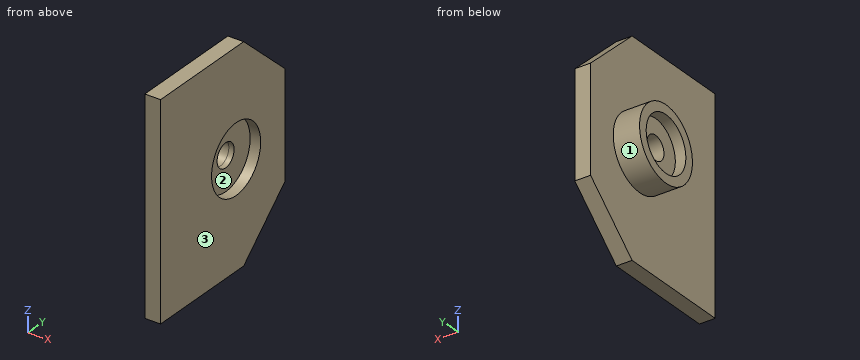
Autodesk Inventor part; units mm, degrees
ref_plane "YZ Plane" through (0, 0, 0) normal (1, 0, 0) x (0, 1, 0)
ref_plane "XZ Plane" through (0, 0, 0) normal (0, 1, 0) x (-1, 0, 0)
ref_plane "XY Plane" through (0, 0, 0) normal (0, 0, 1) x (1, 0, 0)
sketch "Esquisse1" plane through (0, 0, 0) normal (1, 0, 0) x (0, 1, 0)
  circle A0 centre (0, 0) radius 5.25
  circle A1 centre (0, 0) radius 7
  dimension "d0" = 10.5
  dimension "d1" = 14
extrude "Extrusion1" add sketch "Esquisse1" along normal blind 10
sketch "Esquisse2" plane through (10, 0, 0) normal (1, 0, 0) x (0, 0, -1)
  line L0 (20, -20) -> (-20, 20) construction
  line L1 (-20, -20) -> (20, 20) construction
  circle A0 centre (0, 0) radius 17.5 construction
  line L2 (0, 0) -> (0, 13) construction
  line L3 (0, 13) -> (10, 13)
  line L4 (10, 13) -> (-10, 13)
  line L5 (0, 0) -> (0, -20) construction
  line L6 (0, -20) -> (20, -20)
  line L7 (20, -20) -> (-20, -20)
  line L8 (-20, -20) -> (-20, 2)
  line L9 (20, -20) -> (20, 2)
  line L10 (20, 2) -> (10, 13)
  line L11 (-10, 13) -> (-20, 2)
  dimension "d41" = 35
  dimension "d44" = 13
  dimension "d45" = 10
  dimension "d46" = 20
  dimension "d47" = 20
  dimension "d48" = 20
  dimension "d49" = 22
  dimension "d50" = 14.8661
  dimension "d51" = 14.8661
extrude "Extrusion2" add sketch "Esquisse2" along normal blind 3
sketch "Esquisse7" plane through (13, 0, 0) normal (1, 0, 0) x (0, 0, -1)
  circle A0 centre (0, 0) radius 2.25
  dimension "d25" = 4.5
extrude "Extrusion7" cut sketch "Esquisse7" against normal blind 59.75
sketch "Esquisse12" plane through (0, 0, 0) normal (-1, 0, 0) x (0, 0, 1)
  circle A0 centre (0, 0) radius 5.25
  circle A1 centre (0, 0) radius 7
extrude "Extrusion10" cut sketch "Esquisse12" against normal blind 5
sketch "Esquisse13" plane through (13, 0, 0) normal (1, 0, 0) x (0, 0, -1)
  circle A0 centre (0, 0) radius 6.5
  dimension "d52" = 13
extrude "Extrusion11" cut sketch "Esquisse13" against normal blind 2
sketch "Esquisse14" plane through (10, 0, 0) normal (-1, 0, 0) x (0, 0, 1)
  circle A0 centre (0, 0) radius 2.25
  circle A1 centre (0, 0) radius 5.25
extrude "Extrusion12" add sketch "Esquisse14" along normal blind 3
properties part number "percuteur"
Input: part model. Units: mm. Frame: model coordinates. Face numbers are marked on the shaded views. Coordinates: 2 decimals unless noted, no trailing zeros. Write each loop counter-clockwise with the first axis right and the second up, starting at its lowest first coordinate (ties: lowest second). Pieces come first, ordered by that corner, then holes. Notation, with made-up numbers: (-21, -19.5) -> (34, -19.5) arc R18 cw to (34, -12.5) -> close; hole circle Ø10 at (80, 66.25). An arc over 180 degrees is marked (long way). Write each question's results on one line, items separated by ' | '.
Item 1: Section query B-B on x = 12.25. Return loops of the section in (y, z).
Conclusion:
outline: (-20, -20) -> (2, -20) -> (13, -10) -> (13, 10) -> (2, 20) -> (-20, 20) -> close; hole circle Ø13 at (0, 0)
Item 2: Material intervals for probe 1 along Z at (x, y) = (6.3, 0); probe 2 along Y at (x, z) = (12.4, 0); probe 3 along Z at (x, y) = (8.25, 0), sorted ascending.
Conclusion:
probe 1: z = -7 to -5.25, 5.25 to 7 | probe 2: y = -20 to -6.5, 6.5 to 13 | probe 3: z = -7 to -2.25, 2.25 to 7
Item 3: Section query A-A on z = 0. Return loops of the section in (x, y), plus the area to 3 significant figures.
Conclusion:
outline: (5, -7) -> (10, -7) -> (10, -20) -> (13, -20) -> (13, -6.5) -> (11, -6.5) -> (11, -2.25) -> (7, -2.25) -> (7, -5.25) -> (5, -5.25) -> close; (5, 5.25) -> (7, 5.25) -> (7, 2.25) -> (11, 2.25) -> (11, 6.5) -> (13, 6.5) -> (13, 13) -> (10, 13) -> (10, 7) -> (5, 7) -> close | area: 104 mm^2
Item 4: Pin query (flat end, axial travel): pin 1 Ø8 at (y, z) = (2.5, -1) entering from +X; pin 2 Ø3 at (x, z) = (6.5, -0.5) entering from +Y; pin 3 Ø5 at (y, z) = (0, 0) entering from +X; pin 4 Ø5 at (y, z) = (2.5, -1) entering from -X. Return the tip coordinate at first contact, or that it passes through.
Conclusion:
pin 1: stops at x = 13 | pin 2: stops at y = 7 | pin 3: stops at x = 11 | pin 4: stops at x = 7
Item 5: Section query D-D on z = -11. Return loops of the section in (x, y).
Conclusion:
outline: (10, -20) -> (13, -20) -> (13, 11.9) -> (10, 11.9) -> close
Item 6: Section query C-C on y = 0. Return loops of the section in (x, z), plus the area to 3 significant figures.
Conclusion:
outline: (5, -7) -> (10, -7) -> (10, -20) -> (13, -20) -> (13, -6.5) -> (11, -6.5) -> (11, -2.25) -> (7, -2.25) -> (7, -5.25) -> (5, -5.25) -> close; (5, 5.25) -> (7, 5.25) -> (7, 2.25) -> (11, 2.25) -> (11, 6.5) -> (13, 6.5) -> (13, 20) -> (10, 20) -> (10, 7) -> (5, 7) -> close | area: 125 mm^2
Item 7: Mould query, pull axis Y, two halves, no side actions, for the marked faces 1, 2 and 3. Classes: +Y half, -Y half, draft (parallel to the pull), parting line (faces both ways), or undercut.
Conclusion:
face 1: parting line | face 2: undercut | face 3: draft
